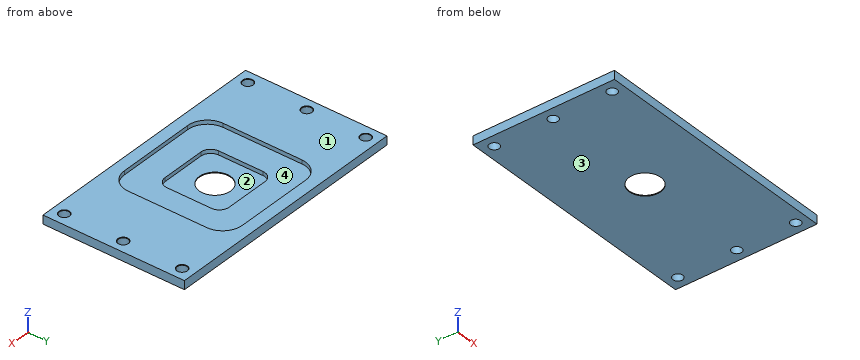
from build123d import *

# Parameters (mm, degrees)
F0_W           = 81.28
F0_H           = 45.72
F1_DEPTH       = 2.794
F3_DEPTH       = 1.27
F4_DEPTH       = 2.54
F2_R           = 5.08
F5_DEPTH       = 2.795
F6_D           = 3.175
F6_CSINK_D     = 3.429
F6_CSINK_ANGLE = 82
F8_D           = 0.01016
F8_DEPTH       = 7.62


with BuildPart() as f1:
    # F0 (on Top) → F1 (new body)
    with BuildSketch(Plane.XY):
        Rectangle(F0_W, F0_H)
    extrude(amount=F1_DEPTH)

    # F2 (on face) → F3 (cut)
    with BuildSketch(Plane.XY.offset(2.794)):
        with BuildLine():
            ThreePointArc((19.05, 12.7), (17.190128, 17.190128), (12.7, 19.05))
            Line((12.7, 19.05), (-12.7, 19.05))
            ThreePointArc((-12.7, 19.05), (-17.190128, 17.190128), (-19.05, 12.7))
            Line((-19.05, 12.7), (-19.05, -12.7))
            ThreePointArc((-19.05, -12.7), (-17.190128, -17.190128), (-12.7, -19.05))
            Line((-12.7, -19.05), (12.7, -19.05))
            ThreePointArc((12.7, -19.05), (17.190128, -17.190128), (19.05, -12.7))
            Line((19.05, -12.7), (19.05, 12.7))
        make_face()
        with BuildLine():
            Line((-7.1755, 10.3505), (7.1755, 10.3505))
            ThreePointArc((7.1755, 10.3505), (9.420564, 9.420564), (10.3505, 7.1755))
            Line((10.3505, 7.1755), (10.3505, -7.1755))
            ThreePointArc((10.3505, -7.1755), (9.420564, -9.420564), (7.1755, -10.3505))
            Line((7.1755, -10.3505), (-7.1755, -10.3505))
            ThreePointArc((-7.1755, -10.3505), (-9.420564, -9.420564), (-10.3505, -7.1755))
            Line((-10.3505, -7.1755), (-10.3505, 7.1755))
            ThreePointArc((-10.3505, 7.1755), (-9.420564, 9.420564), (-7.1755, 10.3505))
        make_face(mode=Mode.SUBTRACT)
    extrude(amount=-F3_DEPTH, mode=Mode.SUBTRACT)

    # F3_face (on face) → F4 (cut)
    with BuildSketch(Plane.XY.offset(2.794)):
        with BuildLine():
            Line((7.1755, 10.3505), (-7.1755, 10.3505))
            ThreePointArc((-7.1755, 10.3505), (-9.420564, 9.420564), (-10.3505, 7.1755))
            Line((-10.3505, 7.1755), (-10.3505, -7.1755))
            ThreePointArc((-10.3505, -7.1755), (-9.420564, -9.420564), (-7.1755, -10.3505))
            Line((-7.1755, -10.3505), (7.1755, -10.3505))
            ThreePointArc((7.1755, -10.3505), (9.420564, -9.420564), (10.3505, -7.1755))
            Line((10.3505, -7.1755), (10.3505, 7.1755))
            ThreePointArc((10.3505, 7.1755), (9.420564, 9.420564), (7.1755, 10.3505))
        make_face()
    extrude(amount=-F4_DEPTH, mode=Mode.SUBTRACT)

    # F2 (on face) → F5 (cut, through all)
    with BuildSketch(Plane.XY.offset(2.794)):
        Circle(F2_R)
    extrude(amount=-F5_DEPTH, mode=Mode.SUBTRACT)

    # F6 (through all)
    with Locations(Plane.XY.offset(2.794)):
        with Locations((-36.83, 19.05), (-36.83, -19.05), (36.83, -19.05), (36.83, 19.05), (-36.83, 0), (36.83, 0)):
            CounterSinkHole(F6_D / 2, F6_CSINK_D / 2, counter_sink_angle=F6_CSINK_ANGLE)

    # F8
    with Locations(Plane.XY.offset(2.794)):
        with Locations((-6.35, 10.541), (0, 10.541), (6.35, 10.541), (6.35, -10.541), (0, -10.541), (-6.35, -10.541)):
            Hole(F8_D / 2, depth=F8_DEPTH)


solid = f1.part
Design review of the part built by this model. Coordinates are the model's own, in mm. Face numbers are marked on the shaded views. A direction names the side the tool comes from. Round coordinates to 2 decimals unless told otherwise and drop trailing zeros. Write each loop counter-clockwise with the first axis right and the second up, starting at its lowest first coordinate (ties: lowest second). Pieces come first, ordered by that corner, then holes. Notation, with made-up numbers: (58.25, -13) - (85.25, -13) arc R32 ccw to (85.25, 26) - close; hole circle Ø4 at (65.25, 46). An arc over 180 degrees is marked (long way). Return JSON: item names as keys, results as strings. Group by question number.
Item 1: We need section D-D on y = 11.5. Write out the cut boundary in (x, z), and give its area (3 significant figures).
Item 2: Machinability: for the marked faces 3 and 4, which of the approach directions +Z, -Z, +X, -X, +Y, -Y give a long, thin tool a straight path to every point of the face, cutting with its end or side? Answer none if there is none.
Item 3: We need section A-A on y = 0. Write out the cut boundary in (x, z).
Item 4: Insertion check: P1, Ø16.5, axis at x = -4, y = 5, coming from the +Z side; P2, Ø1.5, axis at x = -7, y = -1.5, coming from the +Z side. Each pin has a flat end and moves straight along its axis. Give the tip position at first contact, or say it passes through.
Item 5: For probe 1 along Y at (x, z) = (36.83, 1.3); probe 2 along X at (y, z) = (0, 0.65); probe 3 along X at (y, z) = (19, 0.95), list the stretches that pass through material, from the lowest coordinate up. Write a range as [from, to].
Item 6: The part is to be moulded in two halves that separate along X. For the marked faces 1 and 2, say which applies: pulls with the +X half, pulls with the -X half, needs draft (parallel to the pull), parting line crosses it, or undercut.
Item 7: We need section B-B on x = -36.83. Write out the cut boundary in (y, z), and give its area (3 significant figures).
Model answer:
{
 "1": {"outline": "(-40.64, 0) - (40.64, 0) - (40.64, 2.79) - (19.05, 2.79) - (19.05, 1.52) - (-19.05, 1.52) - (-19.05, 2.79) - (-40.64, 2.79) - close", "area": "179 mm²"},
 "2": {"face 3": "-Z, +X, -X, +Y, -Y", "face 4": "+Z"},
 "3": {"outline": "(-40.64, 0) - (-38.42, 0) - (-38.42, 2.65) - (-38.54, 2.79) - (-40.64, 2.79) - close; (-35.24, 0) - (-5.08, 0) - (-5.08, 0.25) - (-10.35, 0.25) - (-10.35, 1.52) - (-19.05, 1.52) - (-19.05, 2.79) - (-35.12, 2.79) - (-35.24, 2.65) - close; (5.08, 0) - (35.24, 0) - (35.24, 2.65) - (35.12, 2.79) - (19.05, 2.79) - (19.05, 1.52) - (10.35, 1.52) - (10.35, 0.25) - (5.08, 0.25) - close; (38.42, 0) - (40.64, 0) - (40.64, 2.79) - (38.54, 2.79) - (38.42, 2.65) - close"},
 "4": {"P1": "stops at z = 1.52", "P2": "stops at z = 0.25"},
 "5": {"probe 1": "y = [-22.86, -20.64], [-17.46, -1.59], [1.59, 17.46], [20.64, 22.86]", "probe 2": "x = [-40.64, -38.42], [-35.24, -10.35], [10.35, 35.24], [38.42, 40.64]", "probe 3": "x = [-40.64, -38.42], [-35.24, 35.24], [38.42, 40.64]"},
 "6": {"face 1": "needs draft", "face 2": "undercut"},
 "7": {"outline": "(-22.86, 0) - (-20.64, 0) - (-20.64, 2.65) - (-20.76, 2.79) - (-22.86, 2.79) - close; (-17.46, 0) - (-1.59, 0) - (-1.59, 2.65) - (-1.71, 2.79) - (-17.34, 2.79) - (-17.46, 2.65) - close; (1.59, 0) - (17.46, 0) - (17.46, 2.65) - (17.34, 2.79) - (1.71, 2.79) - (1.59, 2.65) - close; (20.64, 0) - (22.86, 0) - (22.86, 2.79) - (20.76, 2.79) - (20.64, 2.65) - close", "area": "101 mm²"}
}
